The model under review builds one solid part; all positions refer to its coordinate system, in mm. A direction names the side the tool comes from. Round coordinates to 2 decimals unless told otherwise and drop trailing zeros. Order: outer loops, then holes, each group sorted by start corner. A loop starts at its lowest first (then second) coordinate and runs counter-clockwise, first axis right, second up. Notation, with made-up numbers: (42.5, 74) - (49.5, 74) arc R22 cw to (49.5, 98) - close; hole circle Ø11 at (23, -39.5). An arc over 180 degrees is marked (long way). One line per question, with ' | ' between items. Start each with the question number.
Item 1: Add section A-A on x = 7. State the section outline as (y, z) points.
Item 2: Add section C-C on x = -18. State the section outline as (y, z) points, and give its area (3 significant figures).
Item 3: Insertion check: pin 1 Ø9 at (y, z) = (24, 8) entering from -X; pin 2 Ø4 at (y, z) = (15.5, 11.5) entering from +X; pin 3 Ø3 at (x, z) = (-22, 13) entering from -Y. Each pin has a flat end and moves straight along its axis. Give the tip position at first contact, or say it passes through.
Item 4: Add section D-D on y = 17.5. State the section outline as (x, z) points, and give its area (3 significant figures).
Item 5: Draft analysis for pull direction Z (two halves, no side actions). For faces 6 (the face through (-2, 30, 9)), 7 (the face through (-15, 0, 9)), 8 (the face through (-6, 5, 0)), state which applies: +Z half, -Z half, draft (parallel to the pull), parting line (faces both ways), or undercut.
Item 6: Tool access review of faces 1 (the face through (0, 15, 9)), 2 (the face through (-1, -3, 16)), 3 (the face through (-10, 20, 9)), 4 (the face through (-10, -10, 17)), 5 (the face through (10, 10, 1)): name each direction out of +Z, -Z, +X, -X, +Y, -Y from which nothing blocks a thin tool from reaching the whole face with its end or side.
Item 7: Add section B-B on y = -4.5. State the section outline as (x, z) points.
Item 8: For L1, parallel to Z at x = 1, y = 0; L2, parallel to X at y = 24, z = 7.5; L3, parallel to Y at x = -2, z = 14, list the stretches that pass through material, from the lowest coordinate up. Write a range as [from, to].
from build123d import *

# Parameters (mm, degrees)
F1_DEPTH = 18
F2_W     = 30
F2_H     = 2
F3_DEPTH = 10
F4_W     = 40
F4_H     = 2
F5_DEPTH = 10


with BuildPart() as f1:
    # F0 (on Top) → F1 (new body)
    with BuildSketch(Plane.XY):
        Polygon((0, 30), (-10, 30), (-10, 10), (-30, 10), (-30, 0), (0, 0), align=None)
    extrude(amount=F1_DEPTH)

    # F2 (on face) → F3 (join)
    with BuildSketch(Plane.YZ):
        with Locations((15, 1)):
            Rectangle(F2_W, F2_H)
        with Locations((15, 17)):
            Rectangle(F2_W, F2_H)
    extrude(amount=F3_DEPTH)

    # F4 (on face) → F5 (join)
    with BuildSketch(Plane.XZ):
        with Locations((-10, 17)):
            Rectangle(F4_W, F4_H)
        with Locations((-10, 1)):
            Rectangle(F4_W, F4_H)
    extrude(amount=F5_DEPTH)


solid = f1.part
Determined:
1) outline: (-10, 0) - (30, 0) - (30, 2) - (-10, 2) - close; (-10, 16) - (30, 16) - (30, 18) - (-10, 18) - close
2) outline: (-10, 0) - (10, 0) - (10, 18) - (-10, 18) - (-10, 16) - (0, 16) - (0, 2) - (-10, 2) - close | area: 220 mm2
3) pin 1: x = -10 | pin 2: x = 0 | pin 3: y = 0
4) outline: (-10, 0) - (10, 0) - (10, 2) - (0, 2) - (0, 16) - (10, 16) - (10, 18) - (-10, 18) - close | area: 220 mm2
5) face 6: draft | face 7: undercut | face 8: -Z half
6) face 1: +X, +Y, -Y | face 2: +X, -Y | face 3: +Z, -Z, -X, +Y | face 4: +Z, -Z, +X, -X, -Y | face 5: +Z, -Z, +X, +Y, -Y
7) outline: (-30, 0) - (10, 0) - (10, 2) - (-30, 2) - close; (-30, 16) - (10, 16) - (10, 18) - (-30, 18) - close
8) L1: [0, 2], [16, 18] | L2: [-10, 0] | L3: [0, 30]
